from build123d import *

# Parameters (mm, degrees)
BOSS_EXTRUDE1_DEPTH = 10
CUT_EXTRUDE2_REACH  = 40.351
SKETCH3_R           = 1.375
CUT_EXTRUDE3_REACH  = 40.351
SKETCH4_R           = 1.375


with BuildPart() as part:
    # Sketch2 → Boss-Extrude1 (new body)
    with BuildSketch(Plane(origin=(0, 0, 0), x_dir=(1, 0, 0), z_dir=(0, 1, 0))):
        Polygon((0, 0), (-26.18, 0), (-26.18, 5), (-5, 5), (-5, 26.18), (0, 26.18), align=None)
    extrude(amount=BOSS_EXTRUDE1_DEPTH)

    # Sketch3 → Cut-Extrude2 (cut, up to next)
    with BuildSketch(Plane.XY, mode=Mode.PRIVATE) as cut_extrude2_sk1:
        with Locations((-18.18, 5)):
            Circle(SKETCH3_R)
    cut_extrude2_tool1 = extrude(cut_extrude2_sk1.sketch, amount=-CUT_EXTRUDE2_REACH, mode=Mode.PRIVATE) & part.part
    add(cut_extrude2_tool1.solids().sort_by_distance((-18.18, 5, 0))[0], mode=Mode.SUBTRACT)

    # Sketch4 → Cut-Extrude3 (cut, up to next)
    with BuildSketch(Plane(origin=(0, 0, 0), x_dir=(0, 0, -1), z_dir=(1, 0, 0)), mode=Mode.PRIVATE) as cut_extrude3_sk1:
        with Locations((18.18, 5)):
            Circle(SKETCH4_R)
    cut_extrude3_tool1 = extrude(cut_extrude3_sk1.sketch, amount=-CUT_EXTRUDE3_REACH, mode=Mode.PRIVATE) & part.part
    add(cut_extrude3_tool1.solids().sort_by_distance((0, 5, -18.18))[0], mode=Mode.SUBTRACT)


solid = part.part
Here's how the part is built. I have some questions about the finished solid (model axes, mm). A direction names the side the tool comes from. Coordinates: 2 decimals unless noted, no trailing zeros. Write each loop counter-clockwise with the first axis right and the second up, starting at its lowest first coordinate (ties: lowest second). Pieces come first, ordered by that corner, then holes.
Item 1: I want a section at A-A on z = -18.18. Write out the boundary of the cut face in (x, y) (3 decimals), and give its area (4 significant figures).
Item 2: If we mould it in two halves opening along Y, with no side actions, what happens to faces 1 (the cylindrical face through (-16.868, 5.413, -2.465)), 2 (the flat face through (0, 5, -13)), 3 (the flat face through (-7.1, 0, -4.5))? For each: +Y half, -Y half, draft (parallel to the pull), parting line (faces both ways), or undercut.
Item 3: If I drill on line 1 (Y direction, x = -18.18, z = -2.4) (3 decimals); line 2 (X direction, y = 5.25, z = -15.75), over which ranges is the centre line in solid material (lowest first)?
Item 4: I want a section at C-C on x = -18.18. Write out the boundary of the cut face in (y, z) (3 decimals), and give its area (4 significant figures).
Item 5: Will these pins go through, and if not, where does the flat tip stop? pin 1 (1.5 mm diameter, centred on x = -21.5, y = 7.5, fed in from -Z); pin 2 (6 mm diameter, centred on x = -8.5, z = -23, fed in from +Y) (3 decimals); pin 3 (3 mm diameter, centred on y = 2, z = -9.5, fed in from -X).
Item 6: On a 3-axis mill with a long thin cutter (end or side, diameter ignored), from which of +Z, -Z, +X, -X, +Y, -Y can I reach the whole of each face in a straight line? I mean faces 4 (the flat face through (-7.1, 10, -4.5)), 5 (the flat face through (-5, 5, -15)). Say none if no direction works.
Item 7: I want a section at B-B on y = 5. Write out the boundary of the cut face in (x, z) (3 decimals), and give its area (3 significant figures).
Item 8: I want a section at D-D on z = -2.5. Write out the boundary of the cut face in (x, y) (3 decimals), and give its area (3 significant figures).
Findings below:
1. outline: (-5, 0) - (0, 0) - (0, 3.625) - (-5, 3.625) - close; (-5, 6.375) - (0, 6.375) - (0, 10) - (-5, 10) - close
1. area: 36.25 mm2
2. face 1: undercut
2. face 2: draft
2. face 3: -Y half
3. line 1: y = 0 to 3.625, 6.375 to 10
3. line 2: x = -5 to 0
4. outline: (0, -5) - (3.625, -5) - (3.625, 0) - (0, 0) - close; (6.375, -5) - (10, -5) - (10, 0) - (6.375, 0) - close
4. area: 36.25 mm2
5. pin 1: stops at z = -5
5. pin 2: passes through
5. pin 3: stops at x = -5
6. face 4: +Z, -Z, +X, -X, +Y
6. face 5: -Z, -X, +Y, -Y
7. outline: (-26.18, -5) - (-19.555, -5) - (-19.555, 0) - (-26.18, 0) - close; (-16.805, -5) - (-5, -5) - (-5, -16.805) - (0, -16.805) - (0, 0) - (-16.805, 0) - close; (-5, -26.18) - (0, -26.18) - (0, -19.555) - (-5, -19.555) - close
7. area: 209 mm2
8. outline: (-26.18, 0) - (0, 0) - (0, 10) - (-26.18, 10) - close; hole circle Ø2.75 at (-18.18, 5)
8. area: 256 mm2
